Geometry check sheet. Reference: drawing and pictorial views, mm from the part's lowest x, y, z. Round coordinates to 2 decimals unless told otherwise and drop trailing zeros. Loops run counter-clockwise (first coordinate to the right, second up) from the corner with the lowest first, then second, coordinate; pieces in that order, holes last. Notation, with made-up numbers: (77, 27.25) - (125, 27.25) arc R20 cw to (125, 60.25) - close; hole circle Ø10 at (12.25, -17.5). An arc over 180 degrees is marked (long way). Return JSON: item names as keys, results as strings.
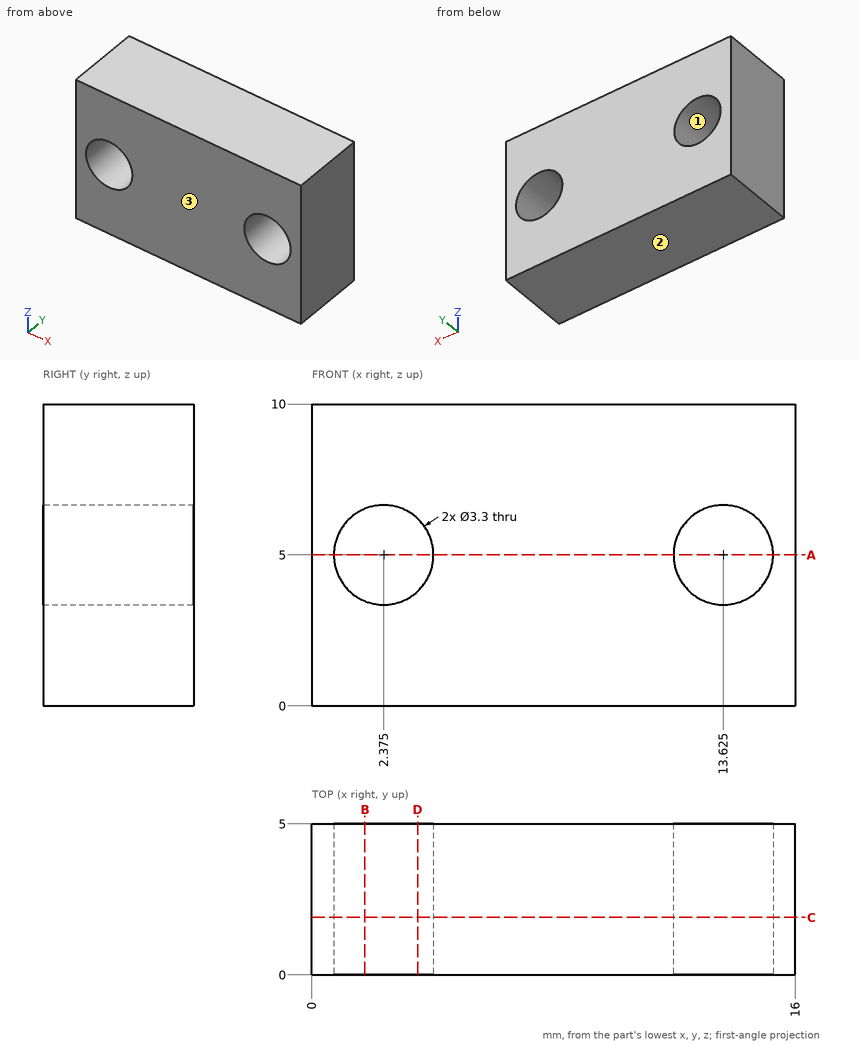
Q1. Scan lines: probe 1 along X at (y, z) = (2.95, 5) (3 decimals); probe 2 along X at (y, z) = (3.7, 6); probe 3 along Z at (x, y) = (14, 3.25). Record each from-to range of solid material in increasing order. Write a range as [from, to].
Answer key:
{"probe 1": "x = [0, 0.725], [4.025, 11.975], [15.275, 16]", "probe 2": "x = [0, 1.06], [3.69, 12.31], [14.94, 16]", "probe 3": "z = [0, 3.39], [6.61, 10]"}
Q2. Draft check along Z on the marked faces 1, 2 and 3. Enter one of: released by +Z, released by -Z, zero draft, split by the parting line, or undercut.
Answer key:
{"face 1": "undercut", "face 2": "released by -Z", "face 3": "zero draft"}
Q3. Sectioned sample at B-B (x = 1.75). Enter the section's corners in (y, z), plus the area to 3 significant figures.
Answer key:
{"outline": "(0, 0) - (5, 0) - (5, 3.47) - (0, 3.47) - close; (0, 6.53) - (5, 6.53) - (5, 10) - (0, 10) - close", "area": "34.7 mm²"}
Q4. Depth check by flat-ended pin: P1, Ø3, axis at x = 2.375, z = 5, coming from the -Y side. Enter the tip coordinate at first touch or a pass-through.
Answer key:
{"P1": "passes through"}
Q5. Sectioned sample at D-D (x = 3.5). Enter the section's corners in (y, z).
Answer key:
{"outline": "(0, 0) - (5, 0) - (5, 3.79) - (0, 3.79) - close; (0, 6.21) - (5, 6.21) - (5, 10) - (0, 10) - close"}
Q6. Sectioned sample at C-C (y = 1.9). Enter the section's corners in (x, z) (3 decimals), plus the area to 3 significant figures.
Answer key:
{"outline": "(0, 0) - (16, 0) - (16, 10) - (0, 10) - close; hole circle Ø3.3 at (2.375, 5); hole circle Ø3.3 at (13.625, 5)", "area": "143 mm²"}
Q7. Sectioned sample at A-A (z = 5). Enter the section's corners in (x, y) (3 decimals), plus the area to 3 significant figures.
Answer key:
{"outline": "(0, 0) - (0.725, 0) - (0.725, 5) - (0, 5) - close; (4.025, 0) - (11.975, 0) - (11.975, 5) - (4.025, 5) - close; (15.275, 0) - (16, 0) - (16, 5) - (15.275, 5) - close", "area": "47.0 mm²"}
